Input: part model. Units: mm. Frame: model coordinates. A direction names the side the tool comes from. Coordinates: 2 decimals unless noted, no trailing zeros.
1) Line query: L1, parallel to Y at x = 3, z = -35.5; L2, parallel to Y at x = 4, z = 19; L3, parallel to Z at x = 16, y = 24.5. Output: solid intervals per line, ascending.
2) Set-up query: faces 1 (the flat face through (-18, 21, -13)), 2 (the flat face through (-50, 5, 1)). Return all of +Z, -Z, +X, -X, +Y, -Y with unobstructed straight access to the full face (end or side cutting, diameter ignored); none if empty.
3) Pin query (flat end, axial travel): pin 1 Ø6 at (x, y) = (-1.5, 23.5) entering from -Z; pin 2 Ø6 at (x, z) = (-34, -12) entering from +Y; pin 3 Ø2 at (y, z) = (13, 0) entering from -X. Return the tip coordinate at first contact, or that it passes through.
from build123d import *

# Parameters (mm, degrees)
SKETCH_1_W      = 100
SKETCH_1_H      = 80
EXTRUDE_1_DEPTH = 10
EXTRUDE_2_DEPTH = 11
EXTRUDE_2_TAPER = 5
EXTRUDE_3_DEPTH = 9
EXTRUDE_3_TAPER = 10


with BuildPart() as part:
    # 스케치1 → 보스-돌출1 (new body)
    with BuildSketch(Plane(origin=(0, 0, 0), x_dir=(1, 0, 0), z_dir=(0, 1, 0))):
        Rectangle(SKETCH_1_W, SKETCH_1_H)
    extrude(amount=EXTRUDE_1_DEPTH)

    # 스케치2 → 보스-돌출2 (add)
    with BuildSketch(Plane(origin=(0, 10, 0), x_dir=(1, 0, 0), z_dir=(0, 1, 0))):
        with BuildLine():
            Line((10, 30), (-41.089791126, 30))
            Line((-41.089791126, 30), (-41.089791126, -30))
            Line((-41.089791126, -30), (10, -30))
            ThreePointArc((10, -30), (40, 0), (10, 30))
        make_face()
    extrude(amount=EXTRUDE_2_DEPTH, taper=EXTRUDE_2_TAPER)

    # 스케치4 → 보스-돌출3 (add)
    with BuildSketch(Plane(origin=(0, 21, 0), x_dir=(1, 0, 0), z_dir=(0, 1, 0))):
        with BuildLine():
            ThreePointArc((-21.764734991, 9.843053917), (-29.999999933, 0.001156755), (-21.767012144, -9.84264538))
            Line((-21.767012144, -9.84264538), (8.542741709, -17.869074273))
            ThreePointArc((8.542741709, -17.869074273), (33.999996077, 0.012209678), (8.51978119, 17.860760459))
            Line((8.51978119, 17.860760459), (-21.764734991, 9.843053917))
        make_face()
    extrude(amount=EXTRUDE_3_DEPTH, taper=EXTRUDE_3_TAPER)


solid = part.part
Answer:
1. L1: y = 0 to 10
1. L2: y = 0 to 21
1. L3: z = -18.36 to 18.36
2. face 1: +Y
2. face 2: +Z, -Z, -X, +Y, -Y
3. pin 1: stops at z = -29.08
3. pin 2: stops at y = 21
3. pin 3: stops at x = -40.91
